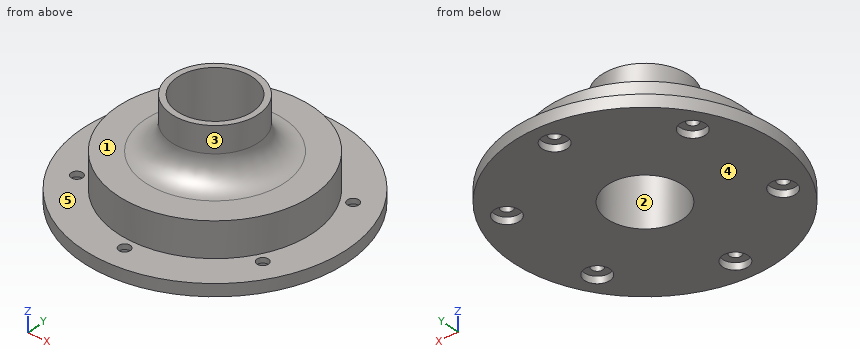
from build123d import *

# Parameters (mm, degrees)
FILLET1_R         = 15
CIRPATTERN1_COUNT = 6


with BuildPart() as part:
    # Sketch1 → Revolve1 (revolve)
    with BuildSketch(Plane(origin=(0, 0, 0), x_dir=(1, 0, 0), z_dir=(0, 1, 0))):
        Polygon((-76.008064516, 0), (-76.008064516, -7), (-56.008064516, -7), (-56.008064516, -27), (-25, -27), (-25, -57), (-21.63, -57), (-21.63, 0), align=None)
    revolve(axis=Axis((0, 0, 0), (0, 0, 1)))

    # Fillet1
    fillet1_edges = [part.edges().sort_by_distance(p)[0] for p in [
        (25, 0, 27),
    ]]
    fillet(fillet1_edges, radius=FILLET1_R)

    # Sketch3 → CBORE for M6 Hex Head Bolt1 (revolve, cut)
    with BuildSketch(Plane(origin=(0, 62, 0), x_dir=(0, 1, 0), z_dir=(1, 0, 0))):
        Polygon((0, 0), (0, 57), (3.3, 57), (3.3, 4), (7.2735, 4), (7.2735, 0.025), (7.2985, 0), align=None)
    cbore_for_m6_hex_head_bolt1 = revolve(axis=Axis((0, 62, -6.35), (0, 0, 1)), mode=Mode.SUBTRACT)

    # CirPattern1: CBORE for M6 Hex Head Bolt1 ×6 about axis
    cirpattern1_axis = Axis((0, 0, 0), (0, 0, 1))
    for i in range(1, CIRPATTERN1_COUNT):
        add(cbore_for_m6_hex_head_bolt1.rotate(cirpattern1_axis, i * 360 / CIRPATTERN1_COUNT), mode=Mode.SUBTRACT)


solid = part.part
Design review of the part built by this model. Coordinates are the model's own, in mm. Face numbers are marked on the shaded views. A direction names the side the tool comes from. Give positions to 0.01 mm unless a question says otherwise; leave off trailing zeros. Write each loop counter-clockwise with the first axis right and the second up, starting at its lowest first coordinate (ties: lowest second). Pieces come first, ordered by that corner, then holes. Notation, with made-up numbers: M -3.5,63 L 32.5,63 A12 ccw 32.5,79 Z; hole C 27.25,-27.75 d9. An arc over 180 degrees is marked long. Answer as a JSON object with one key per item and string values. Group by question number.
1) Mouldability with a two-part tool opening along Y and no side actions: class the marked faces 1, 2 and 3 as released by +Y, released by -Y, zero draft, split by the parting line, or undercut.
2) Tool access review of the marked faces 4 and 5: name each direction out of +Z, -Z, +X, -X, +Y, -Y from which nothing blocks a thin tool from reaching the whole face with its end or side.
3) Clearance check with flat-ended pins moving along their axes: pin 1 Ø23.5 at (x, y) = (0, -62) entering from +Z; pin 2 Ø11.5 at (x, y) = (55, -29.5) entering from -Z; pin 3 Ø4 at (y, z) = (-37.5, 21) entering from -X; pin 4 Ø2 at (x, z) = (-23, 32.5) entering from -Y. State where each tip first meets the part, or that it passes through.
4) We need section B-B (z = 46). Give the boundary of the cut face in (x, y), and give its area (3 significant figures).
5) For line 1 along X through (y, z) = (31, 2.55); line 2 along X through (y, z) = (-31, 6); line 3 along Y through (x, z) = (-53, 6), list the stretches that pass through material, from the lowest coordinate up.
6) We need section C-C (x = 0). Count the separate pieces of the cut face and the enclosed holes in it, and give its area (3 significant figures).
7) We need section A-A (y = 0). Give the boundary of the cut face in (x, z), and give its area (3 significant figures).
Answer key:
{
 "1": {"face 1": "zero draft", "face 2": "undercut", "face 3": "split by the parting line"},
 "2": {"face 4": "-Z, +X, -X, +Y, -Y", "face 5": "+Z"},
 "3": {"pin 1": "stops at z = 27", "pin 2": "stops at z = 0", "pin 3": "stops at x = -43.32", "pin 4": "stops at y = -18.57"},
 "4": {"outline": "C 0,0 d50; hole C 0,0 d43.26", "area": "494 mm²"},
 "5": {"line 1": "x = -69.4 to -60.97, -46.42 to 46.42, 60.97 to 69.4", "line 2": "x = -69.4 to -56.99, -50.39 to 50.39, 56.99 to 69.4", "line 3": "y = -54.48 to -34.23, -27.77 to 27.77, 34.23 to 54.48"},
 "6": {"separate pieces": "4", "enclosed holes": "0", "area": "2,280 mm²"},
 "7": {"outline": "M -76.01,0 L -21.63,0 L -21.63,57 L -25,57 L -25,42 A15 cw -40,27 L -56.01,27 L -56.01,7 L -76.01,7 Z; M 21.63,0 L 76.01,0 L 76.01,7 L 56.01,7 L 56.01,27 L 40,27 A15 cw 25,42 L 25,57 L 21.63,57 Z", "area": "2,440 mm²"}
}
